Could you check a few things on this model? Use its own coordinates, in mm. Face numbers are marked on the shaded views. A direction names the side the tool comes from. Give positions to 0.01 mm unless a question says otherwise; leave off trailing zeros. Order: outer loops, then holes, each group sorted by start corner. A loop starts at its lowest first (then second) coordinate and runs counter-clockwise, first axis right, second up. Notation, with made-up numbers: M 58,19 L 83,19 A20 cw 83,24 Z; hole C -14,23 d4. An arc over 180 degrees is marked long. Answer in a Markdown table with one row per item. Add a question column.
```python
from build123d import *

# Parameters (mm, degrees)
F1_DEPTH = 5
F2_W     = 50
F2_H     = 50
F3_DEPTH = 5
F4_W     = 3.5
F4_H     = 6
F5_DEPTH = 25


with BuildPart() as f1:
    # F0 (on Top) → F1 (new body)
    with BuildSketch(Plane.XY):
        with BuildLine():
            Line((22.44609, 35.041678), (-27.55391, 35.041678))
            ThreePointArc((-27.55391, 35.041678), (-31.089444, 33.577212), (-32.55391, 30.041678))
            Line((-32.55391, 30.041678), (-32.55391, -19.958322))
            ThreePointArc((-32.55391, -19.958322), (-31.089444, -23.493856), (-27.55391, -24.958322))
            Line((-27.55391, -24.958322), (22.44609, -24.958322))
            ThreePointArc((22.44609, -24.958322), (25.981624, -23.493856), (27.44609, -19.958322))
            Line((27.44609, -19.958322), (27.44609, 30.041678))
            ThreePointArc((27.44609, 30.041678), (25.981624, 33.577212), (22.44609, 35.041678))
        make_face()
    extrude(amount=F1_DEPTH)

    # F2 (on face) → F3 (join)
    with BuildSketch(Plane.XY.offset(5)):
        with Locations((-2.55391, 5.041678)):
            Rectangle(F2_W, F2_H)
    extrude(amount=F3_DEPTH)

    # F4 (on face) → F5 (cut)
    with BuildSketch(Plane(origin=(0, 0, 0), x_dir=(1, 0, 0), z_dir=(0, 0, -1))):
        Polygon((-2.38457, -5.041678), (-2.38457, -6.791678), (5.61543, -6.791678), (5.61543, -5.041678), (5.61543, -3.291678), (-2.38457, -3.291678), align=None)
        with Locations((-19.13457, 5.958322)):
            Rectangle(F4_W, F4_H)
        with Locations((-19.13457, -16.041678)):
            Rectangle(F4_W, F4_H)
    extrude(amount=-F5_DEPTH, mode=Mode.SUBTRACT)


solid = f1.part
```
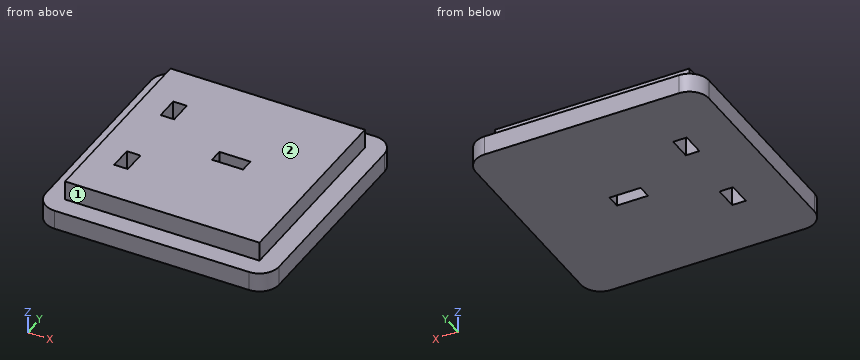
1. Suppose I cut it at B-B on y = 18. List the corners of the cut face in (x, z) for me.
2. Suppose I cut it at D-D on x = -18.5. List the corners of the cut face in (y, z) for me.
3. Suppose I cut it at C-C on z = 8.5. List the corners of the cut face in (x, y) for me.
4. For the marked faces 1 and 2, which set-ups out of +Z, -Z, +X, -X, +Y, -Y let a thin tool reach every point of the face, with its end or its side?
5. If I drill on line 1 along Y through (x, z) = (-19, 1.75); line 2 along Y through (x, z) = (5, 4.25); line 3 along Y through (x, z) = (-18, 6.75), over which ranges is the centre line in solid material (lowest first)? Write a range as [from, to].
6. Will these pins go through, and if not, where does the flat tip stop? P1, Ø1.8, axis at y = 15.5, z = 7.5, coming from the -X side; P2, Ø4, axis at x = -9, z = 8, coming from the +Y side.
7. Suppose I cut it at A-A on x = 0.5. List the corners of the cut face in (y, z) for me.
Findings below:
| question | item | result |
|---|---|---|
| 1 | outline | M -32.55,0 L -20.88,0 L -20.88,10 L -27.55,10 L -27.55,5 L -32.55,5 Z; M -17.38,0 L 27.45,0 L 27.45,5 L 22.45,5 L 22.45,10 L -17.38,10 Z |
| 2 | outline | M -24.96,0 L -8.96,0 L -8.96,10 L -19.96,10 L -19.96,5 L -24.96,5 Z; M -2.96,0 L 13.04,0 L 13.04,10 L -2.96,10 Z; M 19.04,0 L 35.04,0 L 35.04,5 L 30.04,5 L 30.04,10 L 19.04,10 Z |
| 3 | outline | M -27.55,-19.96 L 22.45,-19.96 L 22.45,30.04 L -27.55,30.04 Z; hole M -20.88,-8.96 L -17.38,-8.96 L -17.38,-2.96 L -20.88,-2.96 Z; hole M -20.88,13.04 L -17.38,13.04 L -17.38,19.04 L -20.88,19.04 Z; hole M -2.38,3.29 L 5.62,3.29 L 5.62,6.79 L -2.38,6.79 Z |
| 4 | face 1 | +Z, +X, -X, -Y |
| 4 | face 2 | +Z, +X, -X, +Y, -Y |
| 5 | line 1 | [-24.96, -8.96], [-2.96, 13.04], [19.04, 35.04] |
| 5 | line 2 | [-24.96, 3.29], [6.79, 35.04] |
| 5 | line 3 | [-19.96, -8.96], [-2.96, 13.04], [19.04, 30.04] |
| 6 | P1 | x = -27.55 |
| 6 | P2 | y = 30.04 |
| 7 | outline | M -24.96,0 L 3.29,0 L 3.29,10 L -19.96,10 L -19.96,5 L -24.96,5 Z; M 6.79,0 L 35.04,0 L 35.04,5 L 30.04,5 L 30.04,10 L 6.79,10 Z |
